Can you work these out from the model? Positions are in its coordinate system, mm. A direction names the side the tool comes from. Give positions to 0.01 mm unless a question says otherwise; leave off trailing zeros. Order: outer loops, then holes, each group sorted by start corner. A loop starts at its lowest first (then second) coordinate and runs counter-clockwise, first axis right, second up. Notation, with made-up numbers: (29.5, 53.25) - (62.5, 53.25) arc R24 ccw to (62.5, 81.25) - close; hole circle Ø3 at (50.25, -3.75). An arc over 180 degrees is marked (long way). Return JSON: item names as keys, results as strings.
```python
from build123d import *

# Parameters (mm, degrees)
SKETCH1_R               = 14.35
BOSS_EXTRUDE1_DEPTH     = 7
CUT_EXTRUDE1_DEPTH      = 10
CUT_EXTRUDE2_DEPTH      = 81.06428667
CUT_EXTRUDE2_DEPTH_BACK = 81.06428667
SKETCH3_R               = 3.1
FILLET2_R               = 1
FILLET3_R               = 1
FILLET5_R               = 1
FILLET7_R               = 1


with BuildPart() as part:
    # Sketch1 → Boss-Extrude1 (new body)
    with BuildSketch(Plane(origin=(0, 0, 0), x_dir=(1, 0, 0), z_dir=(0, 1, 0))):
        with BuildLine():
            Line((-45, -18), (45, -18))
            ThreePointArc((45, -18), (52.071067812, -15.071067812), (55, -8))
            Line((55, -8), (55, 8))
            ThreePointArc((55, 8), (52.071067812, 15.071067812), (45, 18))
            Line((45, 18), (-45, 18))
            ThreePointArc((-45, 18), (-52.071067812, 15.071067812), (-55, 8))
            Line((-55, 8), (-55, -8))
            ThreePointArc((-55, -8), (-52.071067812, -15.071067812), (-45, -18))
        make_face()
        with Locations(Location((0, 0, 0), (0, 0, 270))):
            Circle(SKETCH1_R, mode=Mode.SUBTRACT)
    extrude(amount=BOSS_EXTRUDE1_DEPTH)

    # Sketch2 → Cut-Extrude1 (cut)
    with BuildSketch(Plane(origin=(0, 7, 0), x_dir=(1, 0, 0), z_dir=(0, 1, 0))):
        with BuildLine():
            Line((-22.7, 0), (-22.7, 18))
            Line((-22.7, 18), (-47.3, 18))
            Line((-47.3, 18), (-47.3, 0))
            ThreePointArc((-47.3, 0), (-35, -12.3), (-22.7, 0))
        make_face()
    cut_extrude1 = extrude(amount=-CUT_EXTRUDE1_DEPTH, mode=Mode.SUBTRACT)

    # Sketch3 → Cut-Extrude2 (cut, two sides: drawn at the far end of the back side and taken through both)
    with BuildSketch(Plane.ZY.offset(22.7).offset(-CUT_EXTRUDE2_DEPTH_BACK)):
        with Locations((-11.34873736, 3.5)):
            Circle(SKETCH3_R)
    extrude(amount=CUT_EXTRUDE2_DEPTH + CUT_EXTRUDE2_DEPTH_BACK, mode=Mode.SUBTRACT)

    # Fillet2
    fillet2_edges = [part.edges().sort_by_distance(p)[0] for p in [
        (-47.3, 3.5, -17.731906288),
    ]]
    fillet(fillet2_edges, radius=FILLET2_R)

    # Fillet3
    fillet3_edges = [part.edges().sort_by_distance(p)[0] for p in [
        (-22.7, 3.5, -18),
    ]]
    fillet(fillet3_edges, radius=FILLET3_R)

    # Mirror5: Cut-Extrude1 across plane
    add(cut_extrude1.mirror(Plane.ZY), mode=Mode.SUBTRACT)

    # Fillet5
    fillet5_edges = [part.edges().sort_by_distance(p)[0] for p in [
        (47.3, 3.5, -17.731906288),
    ]]
    fillet(fillet5_edges, radius=FILLET5_R)

    # Fillet7
    fillet7_edges = [part.edges().sort_by_distance(p)[0] for p in [
        (22.7, 3.5, -18),
    ]]
    fillet(fillet7_edges, radius=FILLET7_R)


solid = part.part
```
1. Suppose I cut it at C-C (x = 17.5). List the corners of the cut face in (y, z) for me.
Checks:
{"outline": "(0, -18) - (7, -18) - (7, 18) - (0, 18) - close; hole circle Ø6.2 at (3.5, -11.35)"}
2. On a 3-axis mill with a long thin cutter (end or side, diameter ignored), from which of +Z, -Z, +X, -X, +Y, -Y can I reach the whole of each face in a straight line? I mean faces 5 (the face through (-51.095, 2.313, -8.485)), 6 (the face through (47.3, 4, -6)). Say none if no direction works.
Checks:
{"face 5": "+X, -X", "face 6": "-Z, +Y, -Y"}
3. Suppose I cut it at A-A (x = -6). List the corners of the cut face in (y, z) for me.
Checks:
{"outline": "(0, -18) - (7, -18) - (7, -13.04) - (6.1, -13.04) arc R3.1 cw to (0.9, -13.04) - (0, -13.04) - close; (0, 13.04) - (7, 13.04) - (7, 18) - (0, 18) - close"}
4. Thinking about a two-plate mould opening in Z: for faces 1 (the face through (35.27, 3.549, 12.297)), 2 (the face through (51.202, 2.313, -8.485)), 3 (the face through (55, 3, 0)), 4 (the face through (4.31, 3.451, 13.687)), which applies, +Z half, -Z half, draft (parallel to the pull), parting line (faces both ways), or undercut?
Checks:
{"face 1": "-Z half", "face 2": "undercut", "face 3": "draft", "face 4": "undercut"}
5. Suppose I cut it at B-B (y = 3.5). State how many separate pieces and enclosed holes the cut face has, plus the area to 3 significant figures.
Checks:
{"separate pieces": "4", "enclosed holes": "0", "area": "1,600 mm^2"}
6. If I drill on L1, parallel to Z at x = 0, y = 2.5; L2, parallel to X at y = 4.5, z = -7; L3, parallel to Z at x = 8, y = 5.25, over which ranges is the centre line in solid material (lowest first)? Write a range as [from, to].
Checks:
{"L1": "[-18, -14.35], [14.35, 18]", "L2": "[-55, -47.3], [-22.7, -12.53], [12.53, 22.7], [47.3, 55]", "L3": "[-18, -13.91], [11.91, 18]"}
7. Suppose I cut it at D-D (z = 2). List the corners of the cut face in (x, y) for me.
Checks:
{"outline": "(-55, 0) - (-47.14, 0) - (-47.14, 7) - (-55, 7) - close; (-22.86, 0) - (-14.21, 0) - (-14.21, 7) - (-22.86, 7) - close; (14.21, 0) - (22.86, 0) - (22.86, 7) - (14.21, 7) - close; (47.14, 0) - (55, 0) - (55, 7) - (47.14, 7) - close"}
